Can you work these out from the model? Positions are in its coordinate system, mm. Face numbers are marked on the shaded views. Round coordinates to 2 decimals unless told otherwise and drop trailing zeros. Write each loop counter-clockwise with the first axis right and the second up, starting at its lowest first coordinate (ties: lowest second). Pieces come first, ordered by that corner, then holes. Notation, with made-up numbers: M -24.75,77.25 L 23.25,77.25 A17 cw 23.25,85.25 Z; hole C 24,81.25 d7. An arc over 180 degrees is marked long. Answer as a JSON object with one key per item and string values. Group by question number.
1) Suppose I cut it at D-D, the plane x = 2.85. Write out the boundary of the cut face in (y, z), and give its area (3 significant figures).
2) Please list where these lines run through material, in increasing order: L1, parallel to Y at x = 1.1, z = 0; L2, parallel to Z at x = 3, y = -0.25; L3, parallel to Z at x = 1.6, y = 0.75. Write a range as [from, to].
3) I'm going to push flat-ended pins straight in: pin 1 Ø1 at (y, z) = (-4.5, 1) entering from -X; pin 2 Ø2 at (x, y) = (2.5, -3.5) entering from +Z; pin 3 Ø3 at (x, y) = (3, -5) entering from -Z; pin 4 Ø1.5 at (x, z) = (3.5, -5.5) entering from +Y. Where does each tip first touch, or does it pass through?
4) If we mould it in two halves opening along Y, with no side actions, what happens to the marked faces 1, 2 and 3? For each: +Y half, -Y half, draft (parallel to the pull), parting line (faces both ways), or undercut.
5) Suppose I cut it at C-C, the plane x = 0.5. Write out the boundary of the cut face in (y, z).
6) Suppose I cut it at A-A, the plane z = 0. Write out the boundary of the cut face in (x, y).
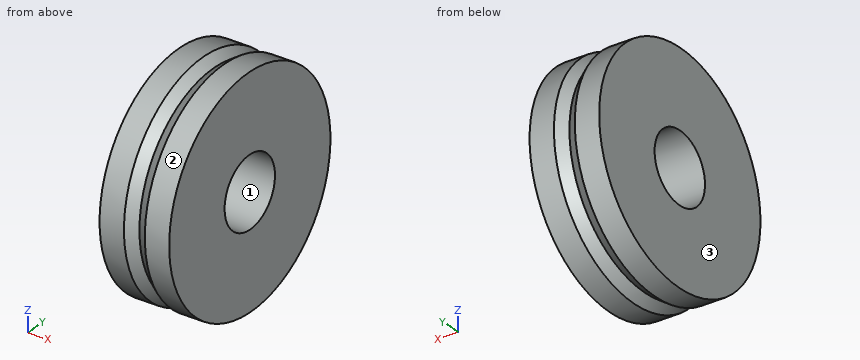
from build123d import *

# Parameters (mm, degrees)
SKETCH1_R           = 8
SKETCH1_R_2         = 2.5
BOSS_EXTRUDE1_DEPTH = 5


with BuildPart() as part:
    # Sketch1 → Boss-Extrude1 (new body)
    with BuildSketch(Plane(origin=(0, 0, 0), x_dir=(0, 0, -1), z_dir=(1, 0, 0))):
        Circle(SKETCH1_R)
        Circle(SKETCH1_R_2, mode=Mode.SUBTRACT)
    extrude(amount=BOSS_EXTRUDE1_DEPTH)

    # Sketch2 → Cut-Revolve1 (revolve, cut)
    with BuildSketch(Plane(origin=(0, 0, 0), x_dir=(1, 0, 0), z_dir=(0, 1, 0))):
        Polygon((1.75, 8), (2.5, 7.5), (3.25, 8), align=None)
    revolve(axis=Axis((0, 0, 0), (1, 0, 0)), mode=Mode.SUBTRACT)


solid = part.part
Results:
{
 "1": {"outline": "C 0,0 d15.47; hole C 0,0 d5", "area": "168 mm^2"},
 "2": {"L1": "[-8, -2.5], [2.5, 8]", "L2": "[-7.83, -2.49], [2.49, 7.83]", "L3": "[-7.96, -2.38], [2.38, 7.96]"},
 "3": {"pin 1": "x = 0", "pin 2": "z = 7.48", "pin 3": "z = -7.18", "pin 4": "y = 6.44"},
 "4": {"face 1": "undercut", "face 2": "parting line", "face 3": "draft"},
 "5": {"outline": "C 0,0 d16; hole C 0,0 d5"},
 "6": {"outline": "M 0,-8 L 1.75,-8 L 2.5,-7.5 L 3.25,-8 L 5,-8 L 5,-2.5 L 0,-2.5 Z; M 0,2.5 L 5,2.5 L 5,8 L 3.25,8 L 2.5,7.5 L 1.75,8 L 0,8 Z"}
}
